Read the model definition and answer for the solid it produces. Units are mm, in the model's axes. A direction names the side the tool comes from. Round coordinates to 2 decimals unless told otherwise and drop trailing zeros. Write each loop counter-clockwise with the first axis right and the second up, starting at its lowest first coordinate (ties: lowest second). Pieces come first, ordered by that corner, then holes. Notation, with made-up numbers: (-31, 12.5) - (8, 12.5) arc R19 cw to (8, 22.5) - close; hole circle Ø5 at (27, 5). An arc over 180 degrees is marked (long way). One line per item, written item: value. Start each with the question number.
(1) Flat-ended cylindrical pins translate along their axes: pin 1 Ø4.5 at (y, z) = (-3, -15.5) entering from -X; pin 2 Ø4 at (y, z) = (-3.5, -12) entering from +X; pin 3 Ø3.5 at (x, y) = (-18.5, -3) entering from +Z (3 decimals). Find the tip coordinate at first contact, or state that the pin passes through.
(2) A cutting plane is placed at A-A, the plane x = 2. Determine the outline of the cut face in (y, z), plus the area to 3 significant figures.
(3) Find the intervals of material crossed by L1, parallel to Z at x = -7, y = -1.5; L2, parallel to Z at x = -17, y = 4.25 (1 decimal); L3, parallel to Z at x = -3.5, y = 1.25, in increasing order.
(4) A cutting plane is placed at B-B, the plane y = 0. State how many separate pieces and enclosed holes the cut face has, plus the area to 3 significant figures.
(5) A cutting plane is placed at D-D, the plane z = -7. Determine the outline of the cut face in (x, y).
(6) The mould has two halves that part along X. Classify faces 1 (the face through (-17, -2, -9.525)), 2 (the face through (-6.803, 0.089, -2.065)), 3 (the face through (-13.813, 0.089, -21.094)), 4 (the face through (25.39, -0.09, -0.75)): +X half, -X half, draft (parallel to the pull), parting line (faces both ways), or undercut.
(7) For faces 5 (the face through (-14.021, 0, -16)), 6 (the face through (-16.5, -0.1, 1.588)), 7 (the face through (-5.9, 0.09, 5.87)), determine the directions among +Z, -Z, +X, -X, +Y, -Y from which every point of the face is accessible in a straight line to the end or side of a thin tool.
from build123d import *

# Parameters (mm, degrees)
F0_R      = 25.4
F1_DEPTH  = 6.35
F3_DEPTH  = 25.4
F5_DEPTH  = 25.4
F6_R      = 1.5875
F8_D      = 3.4544
F10_D     = 5.08
F10_DEPTH = 7.62
F10_TIP   = 1.5261859723
F12_D     = 4.0386
F12_DEPTH = 10.00125
F12_TIP   = 1.213317848


with BuildPart() as f1:
    # F0 (on Front) → F1 (new body, symmetric)
    with BuildSketch(Plane.XZ):
        Circle(F0_R)
    extrude(amount=F1_DEPTH, both=True)

    # F2 (on face) → F3 (cut)
    with BuildSketch(Plane.XZ.offset(6.35)):
        with BuildLine():
            Line((-6.35, -1.5875), (-6.35, 1.5875))
            Line((-6.35, 1.5875), (-25.3503420835, 1.5875))
            ThreePointArc((-25.3503420835, 1.5875), (-25.3875824855, 0.7941382371), (-25.4, 0))
            ThreePointArc((-25.4, 0), (-25.3875824855, -0.7941382371), (-25.3503420835, -1.5875))
            Line((-25.3503420835, -1.5875), (-6.35, -1.5875))
        make_face()
        Polygon((6.35, 6.35), (-6.35, 6.35), (-6.35, 1.5875), (-6.35, -1.5875), (-6.35, -6.35), (6.35, -6.35), align=None)
    extrude(amount=-F3_DEPTH, mode=Mode.SUBTRACT)

    # F4 (on face) → F5 (cut)
    with BuildSketch(Plane.XZ.offset(6.35)):
        with BuildLine():
            Line((-23.5464301965, 9.525), (-14.0214301965, 9.525))
            Line((-14.0214301965, 9.525), (-14.0214301965, 21.1792231974))
            ThreePointArc((-14.0214301965, 21.1792231974), (-19.6670095137, 16.0738525808), (-23.5464301965, 9.525))
        make_face()
        with BuildLine():
            ThreePointArc((-23.5464301965, -9.525), (-19.6670095137, -16.0738525808), (-14.0214301965, -21.1792231974))
            Line((-14.0214301965, -21.1792231974), (-14.0214301965, -9.525))
            Line((-14.0214301965, -9.525), (-23.5464301965, -9.525))
        make_face()
    extrude(amount=-F5_DEPTH, mode=Mode.SUBTRACT)

    # F6
    f6_edges = [f1.edges().sort_by_distance(p)[0] for p in [
        (-23.54643, 0, 9.525),
        (-14.02143, 0, 21.179223),
        (-14.02143, 0, 9.525),
        (-6.35, 0, 6.35),
        (-6.35, 0, 1.5875),
        (-6.35, 0, -1.5875),
        (-6.35, 0, -6.35),
        (6.35, 0, 6.35),
        (6.35, 0, -6.35),
        (-23.54643, 0, -9.525),
        (-14.02143, 0, -9.525),
        (-14.02143, 0, -21.179223),
    ]]
    fillet(f6_edges, radius=F6_R)

    # F8 (through all)
    with Locations(Plane.XZ.offset(6.35)):
        with Locations((-7.2901193866, 17.5999050943), (15.1133811325, 11.5969052226), (15.1133811325, -11.5969052226), (-7.2901193866, -17.5999050943)):
            Hole(F8_D / 2)

    # F10
    with Locations(Plane.XY.offset(9.525)):
        with Locations((-19.0003420835, 0)):
            Hole(F10_D / 2, depth=F10_DEPTH)
            with Locations((0, 0, -(F10_DEPTH + F10_TIP / 2))):  # 118° drill point
                Cone(0, F10_D / 2, F10_TIP, mode=Mode.SUBTRACT)

    # F12
    with Locations(Plane(origin=(0, 0, -9.525), x_dir=(1, 0, 0), z_dir=(0, 0, -1))):
        with Locations((-19.0003420835, 0)):
            Hole(F12_D / 2, depth=F12_DEPTH)
            with Locations((0, 0, -(F12_DEPTH + F12_TIP / 2))):  # 118° drill point
                Cone(0, F12_D / 2, F12_TIP, mode=Mode.SUBTRACT)


solid = f1.part
Here are the results:
1. pin 1: x = -14.02
1. pin 2: x = 23.35
1. pin 3: z = 9.525
2. outline: (-6.35, -25.32) - (6.35, -25.32) - (6.35, -6.35) - (-6.35, -6.35) - close; (-6.35, 6.35) - (6.35, 6.35) - (6.35, 25.32) - (-6.35, 25.32) - close
2. area: 482 mm²
3. L1: -24.42 to -19.3, -15.9 to -1.89, 1.89 to 15.9, 19.3 to 24.42
3. L2: -9.5 to -1.6, 1.6 to 9.5
3. L3: -25.16 to -6.35, 6.35 to 25.16
4. separate pieces: 3
4. enclosed holes: 4
4. area: 1,560 mm²
5. outline: (-24.42, -6.35) - (24.42, -6.35) - (24.42, 6.35) - (-24.42, 6.35) - close; hole circle Ø4.04 at (-19, 0)
6. face 1: draft
6. face 2: undercut
6. face 3: -X half
6. face 4: parting line
7. face 5: -Z, -X, +Y, -Y
7. face 6: -X, +Y, -Y
7. face 7: +Y, -Y
